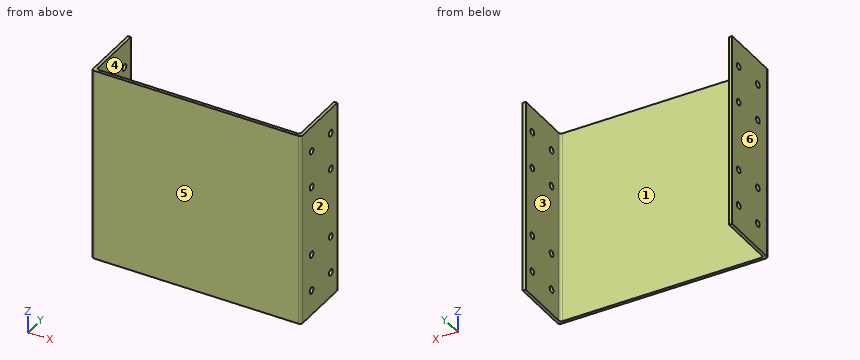
from build123d import *

# Parameters (mm, degrees)
SKETCH2_W           = 171.45
SKETCH2_H           = 158.75
BOSS_EXTRUDE1_DEPTH = 50.8
SKETCH3_W           = 166.37
SKETCH3_H           = 48.26
CUT_EXTRUDE1_DEPTH  = 188.432596218
FILLET1_R           = 2
SKETCH5_R           = 2.5908
SKETCH5_R_2         = 2.5865
CUT_EXTRUDE2_DEPTH  = 196.642871388


with BuildPart() as part:
    # Sketch2 → Boss-Extrude1 (new body)
    with BuildSketch(Plane(origin=(0, 0, 0), x_dir=(1, 0, 0), z_dir=(0, 1, 0))):
        Rectangle(SKETCH2_W, SKETCH2_H)
    extrude(amount=BOSS_EXTRUDE1_DEPTH)

    # Sketch3 → Cut-Extrude1 (cut, through all)
    with BuildSketch(Plane.XY.offset(79.375)):
        with Locations((0, 26.67)):
            Rectangle(SKETCH3_W, SKETCH3_H)
    extrude(amount=-CUT_EXTRUDE1_DEPTH, mode=Mode.SUBTRACT)

    # Fillet1
    fillet1_edges = [part.edges().sort_by_distance(p)[0] for p in [
        (-83.185, 2.54, 0),
        (83.185, 2.54, 0),
        (85.725, 0, 0),
        (-85.725, 0, 0),
    ]]
    fillet(fillet1_edges, radius=FILLET1_R)

    # Sketch5 → Cut-Extrude2 (cut, through all)
    with BuildSketch(Plane(origin=(85.725, 0, 0), x_dir=(0, 0, -1), z_dir=(1, 0, 0))):
        with Locations((-58.83275, 41.7129)):
            Circle(SKETCH5_R)
        with Locations((-58.83275, 14.7)):
            Circle(SKETCH5_R)
        with Locations((58.83275, 41.7129)):
            Circle(SKETCH5_R)
        with Locations((58.83275, 14.7)):
            Circle(SKETCH5_R)
        with Locations((-28.58135, 41.7129)):
            Circle(SKETCH5_R_2)
        with Locations((-28.58135, 14.7)):
            Circle(SKETCH5_R_2)
        with Locations((28.58135, 41.7129)):
            Circle(SKETCH5_R)
        with Locations((28.58135, 14.7)):
            Circle(SKETCH5_R_2)
    extrude(amount=-CUT_EXTRUDE2_DEPTH, mode=Mode.SUBTRACT)


solid = part.part
Design review of the part built by this model. Coordinates are the model's own, in mm. Face numbers are marked on the shaded views. A direction names the side the tool comes from. Coordinates: 2 decimals unless noted, no trailing zeros. Order: outer loops, then holes, each group sorted by start corner. A loop starts at its lowest first (then second) coordinate and runs counter-clockwise, first axis right, second up. Notation, with made-up numbers: M -11.75,22.25 L -7.75,22.25 A19 cw -7.75,41.25 Z; hole C 57.25,26 d1. An arc over 180 degrees is marked long. Use a Markdown table: item, result.
(1) Add section B-B (z = 46). Give the boundary of the cut face in (x, y) (3 decimals).
Worked answers:
| item | result |
|---|---|
| outline | M -85.725,2 A2 ccw -83.725,0 L 83.725,0 A2 ccw 85.725,2 L 85.725,50.8 L 83.185,50.8 L 83.185,4.54 A2 cw 81.185,2.54 L -81.185,2.54 A2 cw -83.185,4.54 L -83.185,50.8 L -85.725,50.8 Z |
(2) Draft analysis for pull direction X (two halves, no side actions). For the marked faces 3, 4, 5 and 6, state which applies: released by +X, released by -X, zero draft, split by the parting line, or undercut.
Worked answers:
| item | result |
|---|---|
| face 3 | undercut |
| face 4 | undercut |
| face 5 | zero draft |
| face 6 | released by -X |
(3) For the marked faces 1 and 2, list the 3-axis set-ups (+Z, -Z, +X, -X, +Y, -Y) from which the entire face can be reached by the end or side of a thin tool; tool diameter is ignored.
Worked answers:
| item | result |
|---|---|
| face 1 | +Z, -Z, +Y |
| face 2 | +Z, -Z, +X, +Y, -Y |
(4) Add section D-D (x = -12). Give the boundary of the cut face in (y, z) (3 decimals).
Worked answers:
| item | result |
|---|---|
| outline | M 0,-79.375 L 2.54,-79.375 L 2.54,79.375 L 0,79.375 Z |
(5) Wall thickness on probe 1 along X at (y, z) = (27, 1) (3 decimals); probe 2 along Y at (x, z) = (20, -23); probe 3 along X at (y, z) = (3, 10) (3 decimals): over which ranges is each line inside the solid? List them lowest first.
Worked answers:
| item | result |
|---|---|
| probe 1 | x = -85.725 to -83.185, 83.185 to 85.725 |
| probe 2 | y = 0 to 2.54 |
| probe 3 | x = -85.725 to -82.461, 82.461 to 85.725 |
(6) Add section C-C (y = 14.7). Count the separate pieces of the cut face and the enclosed holes in it, then the cut area to 3 significant figures.
Worked answers:
| item | result |
|---|---|
| separate pieces | 10 |
| enclosed holes | 0 |
| area | 701 mm2 |
(7) Add section A-A (y = 37). Give the boundary of the cut face in (x, z) (3 decimals), then the cut area to 3 significant figures.
Worked answers:
| item | result |
|---|---|
| outline | M -85.725,-79.375 L -83.185,-79.375 L -83.185,79.375 L -85.725,79.375 Z; M 83.185,-79.375 L 85.725,-79.375 L 85.725,79.375 L 83.185,79.375 Z |
| area | 806 mm2 |
